```python
from build123d import *

# Parameters (mm, degrees)
SKETCH_1_W          = 10
SKETCH_1_H          = 10
SKETCH_1_W_2        = 8
SKETCH_1_H_2        = 8
EXTRUDE_1_DEPTH     = 121
SKETCH_2_R          = 1.5
CUT_EXTRUDE_1_DEPTH = 11
SKETCH_3_R          = 1.5
CUT_EXTRUDE_2_DEPTH = 11


with BuildPart() as part:
    # 草图1 → 拉伸-薄壁1 (new body)
    with BuildSketch(Plane.XY):
        Rectangle(SKETCH_1_W, SKETCH_1_H)
        Rectangle(SKETCH_1_W_2, SKETCH_1_H_2, mode=Mode.SUBTRACT)
    extrude(amount=EXTRUDE_1_DEPTH)

    # 草图2 → 切除-拉伸1 (cut, through all)
    with BuildSketch(Plane(origin=(5, 0, 0), x_dir=(0, 0, -1), z_dir=(1, 0, 0))):
        with Locations((-110.5, 0)):
            Circle(SKETCH_2_R)
        with Locations((-75.5, 0)):
            Circle(SKETCH_2_R)
        with Locations((-45.5, 0)):
            Circle(SKETCH_2_R)
        with Locations((-10.5, 0)):
            Circle(SKETCH_2_R)
    extrude(amount=-CUT_EXTRUDE_1_DEPTH, mode=Mode.SUBTRACT)

    # 草图3 → 切除-拉伸2 (cut, through all)
    with BuildSketch(Plane(origin=(0, 5, 0), x_dir=(1, 0, 0), z_dir=(0, 1, 0))):
        with Locations((0, -60.5)):
            Circle(SKETCH_3_R)
        with Locations((0, -30.5)):
            Circle(SKETCH_3_R)
        with Locations((0, -90.5)):
            Circle(SKETCH_3_R)
    extrude(amount=-CUT_EXTRUDE_2_DEPTH, mode=Mode.SUBTRACT)


solid = part.part
```
Can you work these out from the model? Positions are in its coordinate system, mm. A direction names the side the tool comes from. Give positions to 0.01 mm unless a question says otherwise; leave off trailing zeros. Write each loop counter-clockwise with the first axis right and the second up, starting at its lowest first coordinate (ties: lowest second). Pieces come first, ordered by that corner, then holes. Notation, with made-up numbers: (73, 22.25) -> (99, 22.25) arc R14 ccw to (99, 27.25) -> close; hole circle Ø2 at (29.5, -20.5). An arc over 180 degrees is marked (long way). One line per item, written item: value.
Q1. Imagine slicing it at C-C on z = 87.5. Please give me the cut outline in (x, y), and give its area (3 significant figures).
Results found:
outline: (-5, -5) -> (5, -5) -> (5, 5) -> (-5, 5) -> close; hole (-4, -4) -> (4, -4) -> (4, 4) -> (-4, 4) -> close
area: 36.0 mm^2
Q2. Imagine slicing it at D-D on y = 0. Give the number of separate pieces and of enclosed holes in the cut face, and give its area (3 significant figures).
Results found:
separate pieces: 10
enclosed holes: 0
area: 218 mm^2
Q3. For P1, Ø1.5, axis at x = -2, y = -0.5, coming from the +Z side; P2, Ø4, axis at y = 0, z = 45.5, coming from the -X side, each with a flat end and sliding along its axis, tell me the tip position at first contact or that it passes through.
Results found:
P1: passes through
P2: stops at x = -5
Q4. We'd pull the mould along Y, two halves only. Please class faces 3 (the face through (2, 5, 60)), 4 (the face through (4, 0, 60)), 5 (the face through (-0.195, 4.507, 59.013)): +Y half, -Y half, draft (parallel to the pull), parting line (faces both ways), or undercut.
Results found:
face 3: +Y half
face 4: undercut
face 5: draft
Q5. Which directions (+Z, -Z, +X, -X, +Y, -Y) give clear straight access to the entire face, cutting with the end or side of a thin tool? Please do faces 1 (the face through (-0.195, -4.493, 59.013)), 2 (the face through (-2, 4, 60)).
Results found:
face 1: +Y, -Y
face 2: +Z, -Z
Q6. Imagine slicing it at B-B on z = 45.5. Please give me the cut outline in (x, y).
Results found:
outline: (-5, -5) -> (5, -5) -> (5, -1.5) -> (4, -1.5) -> (4, -4) -> (-4, -4) -> (-4, -1.5) -> (-5, -1.5) -> close; (-5, 1.5) -> (-4, 1.5) -> (-4, 4) -> (4, 4) -> (4, 1.5) -> (5, 1.5) -> (5, 5) -> (-5, 5) -> close
Q7. Imagine slicing it at A-A on x = -2.5. Please give me the cut outline in (y, z).
Results found:
outline: (-5, 0) -> (-4, 0) -> (-4, 121) -> (-5, 121) -> close; (4, 0) -> (5, 0) -> (5, 121) -> (4, 121) -> close
Q8. Please list where these lines run through material, in increasing order: line 1 (Z direction, x = 0, y = -4.5); line 2 (X direction, y = 0.5, z = 97). Write a range as [from, to].
Results found:
line 1: z = [0, 29], [32, 59], [62, 89], [92, 121]
line 2: x = [-5, -4], [4, 5]
